from build123d import *

# Parameters (mm, degrees)
ESQUISSE1_R      = 2.5
EXTRUSION1_DEPTH = 3


with BuildPart() as part:
    # Esquisse1 → Extrusion1 (new body)
    with BuildSketch(Plane(origin=(0, 0, 0), x_dir=(1, 0, 0), z_dir=(0, 1, 0))):
        with BuildLine():
            Line((-64.494367887, 52.858171056), (-99, 26))
            Line((-99, 26), (-105, 26))
            Line((-105, 26), (-105, 39))
            Line((-105, 39), (-126, 39))
            Line((-126, 39), (-126, 26))
            Line((-126, 26), (-132, 26))
            Line((-132, 26), (-132, 54))
            Line((-132, 54), (-102, 54))
            Line((-102, 54), (-102, 95))
            Line((-102, 95), (-84.5, 95))
            Line((-84.5, 95), (-84.5, 90))
            ThreePointArc((-84.5, 90), (-83.035533906, 86.464466094), (-79.5, 85))
            Line((-79.5, 85), (-69.5, 85))
            ThreePointArc((-69.5, 85), (-65.964466094, 86.464466094), (-64.5, 90))
            Line((-64.5, 90), (-64.5, 95))
            Line((-64.5, 95), (64.5, 95))
            Line((64.5, 95), (64.5, 90))
            ThreePointArc((64.5, 90), (65.964466094, 86.464466094), (69.5, 85))
            Line((69.5, 85), (79.5, 85))
            ThreePointArc((79.5, 85), (83.035533906, 86.464466094), (84.5, 90))
            Line((84.5, 90), (84.5, 95))
            Line((84.5, 95), (102, 95))
            Line((102, 95), (102, 54))
            Line((102, 54), (132, 54))
            Line((132, 54), (132, 26))
            Line((132, 26), (126, 26))
            Line((126, 26), (126, 39))
            Line((126, 39), (105, 39))
            Line((105, 39), (105, 26))
            Line((105, 26), (99, 26))
            Line((99, 26), (64.494367887, 52.858171056))
            ThreePointArc((64.494367887, 52.858171056), (0, 75), (-64.494367887, 52.858171056))
        make_face()
        with Locations((-68.793992413, 58.382049127)):
            Circle(ESQUISSE1_R, mode=Mode.SUBTRACT)
        with Locations((68.793992413, 58.382049127)):
            Circle(ESQUISSE1_R, mode=Mode.SUBTRACT)
        with Locations((0, 85)):
            Circle(ESQUISSE1_R, mode=Mode.SUBTRACT)
    extrude(amount=EXTRUSION1_DEPTH)


solid = part.part
Here's how the part is built. I have some questions about the finished solid (model axes, mm). A direction names the side the tool comes from. Give positions to 0.01 mm unless a question says otherwise; leave off trailing zeros. Order: outer loops, then holes, each group sorted by start corner. A loop starts at its lowest first (then second) coordinate and runs counter-clockwise, first axis right, second up. Notation, with made-up numbers: (-30.75, 58.5) -> (28.25, 58.5) arc R29 ccw to (28.25, 84.5) -> close; hole circle Ø3 at (86, -2). An arc over 180 degrees is marked (long way). Use a Markdown table: item, result. Add a question column.
Item 1: If we mould it in two halves opening along Z, with no side actions, what happens to faces 1 (the face through (-66.485, 1.479, -57.425)), 2 (the face through (-83.07, 1.48, -86.5)), 3 (the face through (81.99, 1.48, -39.24))? For each: pulls with the +Z half, pulls with the -Z half, needs draft (parallel to the pull), parting line crosses it, or undercut.
Item 2: Imagine slicing it at A-A on x = 0. Please give me the cut outline in (y, z).
Item 3: Will these pins go through, and if not, where does the flat tip stop? pin 1 (1.5 mm diameter, centred on y = 1, z = -93, fed in from -X); pin 2 (1.5 mm diameter, centred on x = -116, y = 1, fed in from -Z); pin 3 (1.5 mm diameter, centred on x = 76.5, y = 1.5, fed in from -Z); pin 4 (3 mm diameter, centred on x = -68.79, z = -58.38, fed in from -Y).
Item 4: Imagine slicing it at D-D on y = 1.7. Give the number of separate pieces and of enclosed holes in the cut face, plus the area to 3 significant figures.
Item 5: For faces 4 (the face through (65.93, 1.48, -86.5)), 5 (the face through (-81.506, 1.479, -39.617)), 6 (the face through (66.81, 1.48, -56.86)), which set-ups out of +Z, -Z, +X, -X, +Y, -Y let a thin tool reach every point of the face, with its end or its side?
Item 6: Imagine slicing it at B-B on z = -33. Please give me the cut outline in (x, y).
Item 7: Imagine slicing it at C-C on z = -47. Please give me the cut outline in (x, y).
Item 8: I need wall thicknesses on line 1 (X direction, y = 0.9, z = -89.5); line 2 (X direction, y = 0.7, z = -51.5); line 3 (Z direction, x = 0, y = 1.65). Which ranges of each line are inside material? Lowest first, please.
Data:
| question | item | result |
|---|---|---|
| 1 | face 1 | undercut |
| 1 | face 2 | pulls with the -Z half |
| 1 | face 3 | pulls with the +Z half |
| 2 | outline | (0, -95) -> (3, -95) -> (3, -87.5) -> (0, -87.5) -> close; (0, -82.5) -> (3, -82.5) -> (3, -75) -> (0, -75) -> close |
| 3 | pin 1 | stops at x = -102 |
| 3 | pin 2 | stops at z = -54 |
| 3 | pin 3 | stops at z = -85 |
| 3 | pin 4 | passes through |
| 4 | separate pieces | 1 |
| 4 | enclosed holes | 3 |
| 4 | area | 8,430 mm² |
| 5 | face 4 | -Z, +Y, -Y |
| 5 | face 5 | +Z, +Y, -Y |
| 5 | face 6 | +Y, -Y |
| 6 | outline | (-132, 0) -> (-126, 0) -> (-126, 3) -> (-132, 3) -> close; (-105, 0) -> (-90.01, 0) -> (-90.01, 3) -> (-105, 3) -> close; (90.01, 0) -> (105, 0) -> (105, 3) -> (90.01, 3) -> close; (126, 0) -> (132, 0) -> (132, 3) -> (126, 3) -> close |
| 7 | outline | (-132, 0) -> (-72.02, 0) -> (-72.02, 3) -> (-132, 3) -> close; (72.02, 0) -> (132, 0) -> (132, 3) -> (72.02, 3) -> close |
| 8 | line 1 | x = -102 to -84.47, -64.53 to 64.53, 84.47 to 102 |
| 8 | line 2 | x = -132 to -66.24, 66.24 to 132 |
| 8 | line 3 | z = -95 to -87.5, -82.5 to -75 |
